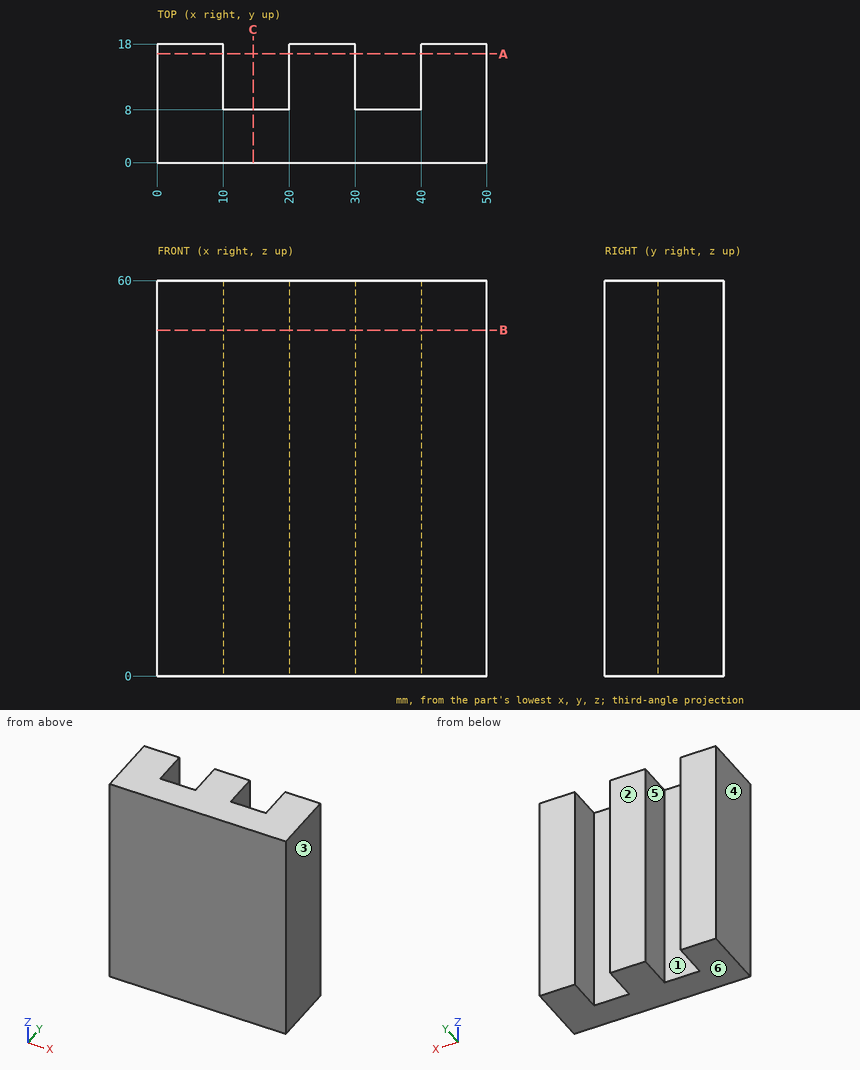
Geometry: see drawing. Coordinates: mm, zero at the bounding-box minimum. A direction names the side the tool comes from. Round coordinates to 2 decimals unless told otherwise and drop trailing zeros. Write each loop counter-clockwise with the first axis right and the second up, starting at its lowest first coordinate (ties: lowest second). Pieces come first, ordered by that corner, then holes.
1) Ray query, L1, parallel to X at y = 17.25, z = 20; L2, parallel to Y at x = 13.5, z = 9. Return the intervals inside material, ascending.
2) Cut plane A-A (y = 16.5). Return the cut outline in (x, z).
3) Draft query along X for the marked faces 1, 2, 3 and 4. Return one class per face: pulls with the +X half, pulls with the -X half, needs draft (parallel to the pull), parting line crosses it, or undercut.
4) Contact query for a flat-ended pin moving along its axis: P1, Ø3, axis at x = 34, z = 36.5, coming from the +Y side. Output: stop coordinate, or through.
5) Cut plane C-C (x = 14.5). Return the cut outline in (y, z).
6) Cut plane B-B (z = 52.5). Return the cut outline in (x, y).
7) Reachability of the marked faces 5 and 6 from +Z, -Z, +X, -X, +Y, -Y: full face, straight path, thin tool, end or side. Return the list, or none.
Geometry says:
1. L1: x = 0 to 10, 20 to 30, 40 to 50
1. L2: y = 0 to 8
2. outline: (0, 0) - (10, 0) - (10, 60) - (0, 60) - close; (20, 0) - (30, 0) - (30, 60) - (20, 60) - close; (40, 0) - (50, 0) - (50, 60) - (40, 60) - close
3. face 1: undercut
3. face 2: needs draft
3. face 3: pulls with the +X half
3. face 4: pulls with the -X half
4. P1: stops at y = 8
5. outline: (0, 0) - (8, 0) - (8, 60) - (0, 60) - close
6. outline: (0, 0) - (50, 0) - (50, 18) - (40, 18) - (40, 8) - (30, 8) - (30, 18) - (20, 18) - (20, 8) - (10, 8) - (10, 18) - (0, 18) - close
7. face 5: +Z, -Z, +Y
7. face 6: -Z, +X, -X, +Y, -Y
